from build123d import *

# Parameters (mm, degrees)
EXTRUDE_1_DEPTH     = 58.89737674
EXTRUDE_START       = 38.399597665
EXTRUDE_2_DEPTH     = 38.399597665
EXTRUDE_3_REACH     = 66.893
SKETCH_3_W          = 44.2
SKETCH_3_H          = 3
EXTRUDE_4_REACH     = 66.893
SKETCH_4_W          = 44.2
SKETCH_4_H          = 3
CUT_EXTRUDE_START   = -77.29697691
CUT_EXTRUDE_1_DEPTH = 77.29697691
SKETCH_6_W          = 10.588620777
SKETCH_6_H          = 6.5
CUT_EXTRUDE_2_DEPTH = 3
EXTRUDE_START_2     = 15
EXTRUDE_5_DEPTH     = 15


with BuildPart() as part:
    # 草图1 → 凸台-拉伸1 (new body)
    with BuildSketch(Plane(origin=(0, 0, 0), x_dir=(1, 0, 0), z_dir=(0, 1, 0))):
        with BuildLine():
            Line((21.346642729, -10.719560241), (16.852020459, -16.362765964))
            ThreePointArc((16.852020459, -16.362765964), (15.807857901, -17.196247295), (14.505374257, -17.493741725))
            Line((14.505374257, -17.493741725), (-14.505381202, -17.493741725))
            ThreePointArc((-14.505381202, -17.493741725), (-15.807864846, -17.196247295), (-16.852027404, -16.362765964))
            Line((-16.852027404, -16.362765964), (-21.346649674, -10.719560241))
            ThreePointArc((-21.346649674, -10.719560241), (-21.831958504, -9.840501001), (-22.000003473, -8.850536003))
            Line((-22.000003473, -8.850536003), (-23.000003473, -8.850536003))
            ThreePointArc((-23.000003473, -8.850536003), (-23.707110254, -8.557642784), (-24.000003473, -7.850536003))
            Line((-24.000003473, -7.850536003), (-24.000003473, -1.349569462))
            ThreePointArc((-24.000003473, -1.349569462), (-23.707110254, -0.642462681), (-23.000003473, -0.349569462))
            Line((-23.000003473, -0.349569462), (-22.100003473, -0.349569462))
            Line((-22.100003473, -0.349569462), (-22.100003473, -4.600052733))
            Line((-22.100003473, -4.600052733), (-22.000003473, -4.600052733))
            Line((-22.000003473, -4.600052733), (-20.000003473, -4.600052733))
            Line((-20.000003473, -4.600052733), (-20.000003473, -9.200105465))
            Line((-20.000003473, -9.200105465), (-14.987335304, -15.493741725))
            Line((-14.987335304, -15.493741725), (14.987328359, -15.493741725))
            Line((14.987328359, -15.493741725), (19.999996527, -9.200105465))
            Line((19.999996527, -9.200105465), (19.999996527, -4.600052733))
            Line((19.999996527, -4.600052733), (21.999996527, -4.600052733))
            Line((21.999996527, -4.600052733), (22.099996527, -4.600052733))
            Line((22.099996527, -4.600052733), (22.099996527, -0.349569462))
            Line((22.099996527, -0.349569462), (22.999996527, -0.349569462))
            ThreePointArc((22.999996527, -0.349569462), (23.707103309, -0.642462681), (23.999996527, -1.349569462))
            Line((23.999996527, -1.349569462), (23.999996527, -7.850536003))
            ThreePointArc((23.999996527, -7.850536003), (23.707103309, -8.557642784), (22.999996527, -8.850536003))
            Line((22.999996527, -8.850536003), (21.999996527, -8.850536003))
            ThreePointArc((21.999996527, -8.850536003), (21.831951559, -9.840501001), (21.346642729, -10.719560241))
        make_face()
    extrude(amount=EXTRUDE_1_DEPTH)

    # 草图2 → 凸台-拉伸2 (add)
    with BuildSketch(Plane.XZ.offset(EXTRUDE_START)):
        with BuildLine():
            Line((22.999996527, 8.850536003), (21.999996527, 8.850536003))
            ThreePointArc((21.999996527, 8.850536003), (21.831951559, 9.840501001), (21.346642729, 10.719560241))
            Line((21.346642729, 10.719560241), (16.852020459, 16.362765964))
            ThreePointArc((16.852020459, 16.362765964), (15.807857901, 17.196247295), (14.505374257, 17.493741725))
            Line((14.505374257, 17.493741725), (-14.505381202, 17.493741725))
            ThreePointArc((-14.505381202, 17.493741725), (-15.807864846, 17.196247295), (-16.852027404, 16.362765964))
            Line((-16.852027404, 16.362765964), (-21.346649674, 10.719560241))
            ThreePointArc((-21.346649674, 10.719560241), (-21.831958504, 9.840501001), (-22.000003473, 8.850536003))
            Line((-22.000003473, 8.850536003), (-23.000003473, 8.850536003))
            ThreePointArc((-23.000003473, 8.850536003), (-23.707110254, 8.557642784), (-24.000003473, 7.850536003))
            Line((-24.000003473, 7.850536003), (-24.000003473, 1.349569462))
            ThreePointArc((-24.000003473, 1.349569462), (-23.707110254, 0.642462681), (-23.000003473, 0.349569462))
            Line((-23.000003473, 0.349569462), (-22.100003473, 0.349569462))
            Line((-22.100003473, 0.349569462), (-22.100003473, 4.600052733))
            Line((-22.100003473, 4.600052733), (-20.000003473, 4.600052733))
            Line((-20.000003473, 4.600052733), (-20.000003473, 9.200105465))
            Line((-20.000003473, 9.200105465), (-14.987335304, 15.493741725))
            Line((-14.987335304, 15.493741725), (14.987328359, 15.493741725))
            Line((14.987328359, 15.493741725), (19.999996527, 9.200105465))
            Line((19.999996527, 9.200105465), (19.999996527, 4.600052733))
            Line((19.999996527, 4.600052733), (22.099996527, 4.600052733))
            Line((22.099996527, 4.600052733), (22.099996527, 0.349569462))
            Line((22.099996527, 0.349569462), (22.999996527, 0.349569462))
            ThreePointArc((22.999996527, 0.349569462), (23.707103309, 0.642462681), (23.999996527, 1.349569462))
            Line((23.999996527, 1.349569462), (23.999996527, 7.850536003))
            ThreePointArc((23.999996527, 7.850536003), (23.707103309, 8.557642784), (22.999996527, 8.850536003))
        make_face()
    extrude(amount=-EXTRUDE_2_DEPTH)

    # 凸台-拉伸3: up to this face of the body (flat: up to its plane)
    extrude_3_end = Plane(part.part.faces().sort_by_distance((-3.473e-06, 10.248889538, 17.493741725))[0])
    # 草图3 → 凸台-拉伸3 (add, up to the picked face)
    with BuildSketch(Plane(origin=(0, 0, 4.600052733), x_dir=(-1, 0, 0), z_dir=(0, 0, -1)), mode=Mode.PRIVATE) as extrude_3_sk1:
        with Locations((3.473e-06, -36.899597665)):
            Rectangle(SKETCH_3_W, SKETCH_3_H)
    extrude_3_tool1 = split(extrude(extrude_3_sk1.sketch, amount=-EXTRUDE_3_REACH, mode=Mode.PRIVATE), bisect_by=extrude_3_end, keep=Keep.BOTH, mode=Mode.PRIVATE)
    add(extrude_3_tool1.solids().sort_by(Axis((-3e-06, -36.899598, 4.600053), (0, 0, 1)))[0])

    # 凸台-拉伸4: up to this face of the body (flat: up to its plane)
    extrude_4_end = Plane(part.part.faces().sort_by_distance((-3.473e-06, 9.499837909, 17.493741725))[0])
    # 草图4 → 凸台-拉伸4 (add, up to the picked face)
    with BuildSketch(Plane(origin=(0, 0, 4.600052733), x_dir=(-1, 0, 0), z_dir=(0, 0, -1)), mode=Mode.PRIVATE) as extrude_4_sk1:
        with Locations((3.473e-06, 37.397379245)):
            Rectangle(SKETCH_4_W, SKETCH_4_H)
    extrude_4_tool1 = split(extrude(extrude_4_sk1.sketch, amount=-EXTRUDE_4_REACH, mode=Mode.PRIVATE), bisect_by=extrude_4_end, keep=Keep.BOTH, mode=Mode.PRIVATE)
    add(extrude_4_tool1.solids().sort_by(Axis((-3e-06, 37.397379, 4.600053), (0, 0, 1)))[0])

    # 草图5 → 切除-拉伸1 (cut)
    with BuildSketch(Plane(origin=(0, 38.897379245, 0), x_dir=(1, 0, 0), z_dir=(0, 1, 0)).offset(CUT_EXTRUDE_START)):
        with BuildLine():
            Line((-22.100003473, -8.850536003), (-22.100003473, -17.493741725))
            Line((-22.100003473, -17.493741725), (-14.505381202, -17.493741725))
            ThreePointArc((-14.505381202, -17.493741725), (-15.807864846, -17.196247295), (-16.852027404, -16.362765964))
            Line((-16.852027404, -16.362765964), (-21.346649674, -10.719560241))
            ThreePointArc((-21.346649674, -10.719560241), (-21.831958504, -9.840501001), (-22.000003473, -8.850536003))
            Line((-22.000003473, -8.850536003), (-22.100003473, -8.850536003))
        make_face()
        with BuildLine():
            Line((14.505374257, -17.493741725), (22.099996527, -17.493741725))
            Line((22.099996527, -17.493741725), (22.099996527, -8.850536003))
            Line((22.099996527, -8.850536003), (21.999996527, -8.850536003))
            ThreePointArc((21.999996527, -8.850536003), (21.831951559, -9.840501001), (21.346642729, -10.719560241))
            Line((21.346642729, -10.719560241), (16.852020459, -16.362765964))
            ThreePointArc((16.852020459, -16.362765964), (15.807857901, -17.196247295), (14.505374257, -17.493741725))
        make_face()
    extrude(amount=CUT_EXTRUDE_1_DEPTH, mode=Mode.SUBTRACT)

    # 草图6 → 切除-拉伸2 (cut)
    with BuildSketch(Plane(origin=(0, 38.897379245, 0), x_dir=(1, 0, 0), z_dir=(0, 1, 0))):
        with Locations((-3.3e-06, -10.750052671)):
            Rectangle(SKETCH_6_W, SKETCH_6_H)
    extrude(amount=-CUT_EXTRUDE_2_DEPTH, mode=Mode.SUBTRACT)

    # 草图7 → 凸台-拉伸5 (add)
    with BuildSketch(Plane(origin=(0, -38.399597665, 0), x_dir=(-1, 0, 0), z_dir=(0, -1, 0)).offset(EXTRUDE_START_2)):
        with BuildLine():
            Line((20.000003473, -4.600052733), (20.000003473, -9.200105465))
            Line((20.000003473, -9.200105465), (14.987335304, -15.493741725))
            Line((14.987335304, -15.493741725), (-14.987328359, -15.493741725))
            Line((-14.987328359, -15.493741725), (-19.999996527, -9.200105465))
            Line((-19.999996527, -9.200105465), (-19.999996527, -4.600052733))
            Line((-19.999996527, -4.600052733), (-21.999996527, -4.600052733))
            Line((-21.999996527, -4.600052733), (-22.099996527, -4.600052733))
            Line((-22.099996527, -4.600052733), (-22.099996527, -0.349569462))
            Line((-22.099996527, -0.349569462), (-22.999996527, -0.349569462))
            ThreePointArc((-22.999996527, -0.349569462), (-23.707103309, -0.642462681), (-23.999996527, -1.349569462))
            Line((-23.999996527, -1.349569462), (-23.999996527, -7.850536003))
            ThreePointArc((-23.999996527, -7.850536003), (-23.707103309, -8.557642784), (-22.999996527, -8.850536003))
            Line((-22.999996527, -8.850536003), (-21.999996527, -8.850536003))
            ThreePointArc((-21.999996527, -8.850536003), (-21.831951559, -9.840501001), (-21.346642729, -10.719560241))
            Line((-21.346642729, -10.719560241), (-16.852020459, -16.362765964))
            ThreePointArc((-16.852020459, -16.362765964), (-15.807857901, -17.196247295), (-14.505374257, -17.493741725))
            Line((-14.505374257, -17.493741725), (14.505381202, -17.493741725))
            ThreePointArc((14.505381202, -17.493741725), (15.807864846, -17.196247295), (16.852027404, -16.362765964))
            Line((16.852027404, -16.362765964), (21.346649674, -10.719560241))
            ThreePointArc((21.346649674, -10.719560241), (21.831958504, -9.840501001), (22.000003473, -8.850536003))
            Line((22.000003473, -8.850536003), (23.000003473, -8.850536003))
            ThreePointArc((23.000003473, -8.850536003), (23.707110254, -8.557642784), (24.000003473, -7.850536003))
            Line((24.000003473, -7.850536003), (24.000003473, -1.349569462))
            ThreePointArc((24.000003473, -1.349569462), (23.707110254, -0.642462681), (23.000003473, -0.349569462))
            Line((23.000003473, -0.349569462), (22.100003473, -0.349569462))
            Line((22.100003473, -0.349569462), (22.100003473, -4.600052733))
            Line((22.100003473, -4.600052733), (22.000003473, -4.600052733))
            Line((22.000003473, -4.600052733), (20.000003473, -4.600052733))
        make_face()
    extrude(amount=-EXTRUDE_5_DEPTH)

    # 草图8 → 切除-旋转1 (revolve, cut)
    with BuildSketch(Plane(origin=(0, 0, 0), x_dir=(0, 0, -1), z_dir=(1, 0, 0))):
        Polygon((-9.89924439, -38.299597665), (-20.291549236, -44.299597665), (-20.291549236, -55.801852499), (11.09144377, -55.801852499), (11.09144377, -44.299597665), (0.699138925, -38.299597665), align=None)
    revolve(axis=Axis((0, -108.399597665, 9.89924439), (0, 0, -1)), mode=Mode.SUBTRACT)


solid = part.part
For this review, take the finished solid that the model builds, in its own axes (mm). A direction names the side the tool comes from. Give positions to 0.01 mm unless a question says otherwise; leave off trailing zeros. Loops run counter-clockwise (first coordinate to the right, second up) from the corner with the lowest first, then second, coordinate; pieces in that order, holes last.
Item 1: Take a section at A-A, the plane y = -14.5. State the section outline as (x, z) points, and give its area (3 significant figures).
Item 2: For line 1 along X through (y, z) = (-10, 6); line 2 along Y through (x, z) = (-13.5, 7); line 3 along X through (y, z) = (0, 2.25), list the stretches that pass through material, from the lowest coordinate up.
Item 3: Take a section at B-B, the plane z = 6.5. State the section outline as (x, y) points.
Item 4: Draft analysis for pull direction Y (two halves, no side actions). For faces 6 (the flat face through (0, -35.4, 10)), 7 (the flat face through (17.46, -40.31, 12.39)), 8 (the flat face through (0, -38.4, 11)), state which applies: +Y half, -Y half, draft (parallel to the pull), parting line (faces both ways), or undercut.
Item 5: Tool access review of faces 1 (the cylindrical face through (-22.27, -41.93, 5.19)), 2 (the flat face through (20, 49, 7)), 3 (the flat face through (5.294, 37, 11)), 4 (the flat face through (22.1, 8, 3)), 5 (the flat face through (17.46, -0.25, 12.39)): name each direction out of +Z, -Z, +X, -X, +Y, -Y from which nothing blocks a thin tool from reaching the whole face with its end or side.
Item 6: Insertion check: pin 1 (0.9 mm diameter, centred on y = 37.5, z = 11.5, fed in from +X); pin 2 (8.5 mm diameter, centred on x = 4.5, z = 12.5, fed in from -Y); pin 3 (5 mm diameter, centred on x = -14, z = 7, fed in from -Y). Each pin has a flat end and moves straight along its axis. Give the tip position at first contact, or say it passes through.
Calculated:
1. outline: (-24, 1.35) arc R1 ccw to (-23, 0.35) - (-22.1, 0.35) - (-22.1, 4.6) - (-20, 4.6) - (-20, 9.2) - (-14.99, 15.49) - (14.99, 15.49) - (20, 9.2) - (20, 4.6) - (22.1, 4.6) - (22.1, 0.35) - (23, 0.35) arc R1 ccw to (24, 1.35) - (24, 7.85) arc R1 ccw to (23, 8.85) - (22, 8.85) arc R3 ccw to (21.35, 10.72) - (16.85, 16.36) arc R3 ccw to (14.51, 17.49) - (-14.51, 17.49) arc R3 ccw to (-16.85, 16.36) - (-21.35, 10.72) arc R3 ccw to (-22, 8.85) - (-23, 8.85) arc R1 ccw to (-24, 7.85) - close
1. area: 149 mm2
2. line 1: x = -24 to -20, 20 to 24
2. line 2: y = -38.4 to -35.4, 35.9 to 38.9
2. line 3: x = -24 to -22.1, 22.1 to 24
3. outline: (-24, -42.54) arc R70.1 cw to (-20, -41.21) - (-20, -38.4) - (-3.74, -38.4) arc R70.1 cw to (3.74, -38.4) - (20, -38.4) - (20, -41.21) arc R70.1 cw to (24, -42.54) - (24, 58.9) - (20, 58.9) - (20, 38.9) - (-20, 38.9) - (-20, 58.9) - (-24, 58.9) - close; hole (-20, -35.4) - (20, -35.4) - (20, 35.9) - (-20, 35.9) - close
4. face 6: undercut
4. face 7: draft
4. face 8: -Y half
5. face 1: -Z, -Y
5. face 2: -Z, +Y
5. face 3: +Y
5. face 4: -Z, +Y, -Y
5. face 5: -Z
6. pin 1: stops at x = 21.08
6. pin 2: stops at y = -42.43
6. pin 3: stops at y = -38.4
